Can you work these out from the model? Positions are in its coordinate system, mm. Face numbers are marked on the shaded views. A direction names the side the tool comes from. Give positions to 0.01 mm unless a question says otherwise; leave off trailing zeros. Order: outer loops, then holes, each group sorted by start corner. A loop starts at its lowest first (then second) coordinate and runs counter-clockwise, first axis right, second up. Notation, with made-up numbers: (-14.75, 4.25) - (18.25, 4.25) arc R21 ccw to (18.25, 32.25) - close; hole circle Ø2 at (77, 52.5). An arc over 180 degrees is marked (long way). Answer as a JSON object with one key per item and string values.
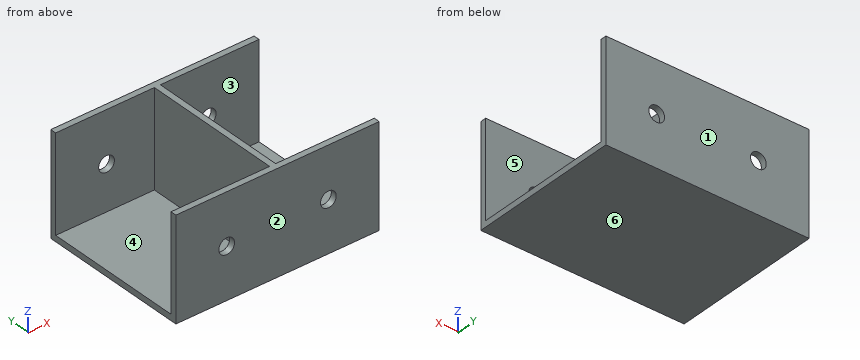
```python
from build123d import *

# Parameters (mm, degrees)
SKETCH1_W           = 101.6
SKETCH1_H           = 76.2
BOSS_EXTRUDE1_DEPTH = 50.8
SKETCH3_W           = 49.3
SKETCH3_H           = 70.2
CUT_EXTRUDE1_DEPTH  = 47.8
SKETCH4_R           = 3.937
CUT_EXTRUDE3_DEPTH  = 50.8


with BuildPart() as part:
    # Sketch1 → Boss-Extrude1 (new body)
    with BuildSketch(Plane.XY):
        Rectangle(SKETCH1_W, SKETCH1_H)
    extrude(amount=BOSS_EXTRUDE1_DEPTH)

    # Sketch3 → Cut-Extrude1 (cut)
    with BuildSketch(Plane.XY.offset(50.8)):
        with Locations((-26.15, 0)):
            Rectangle(SKETCH3_W, SKETCH3_H)
        with Locations((26.15, 0)):
            Rectangle(SKETCH3_W, SKETCH3_H)
    extrude(amount=-CUT_EXTRUDE1_DEPTH, mode=Mode.SUBTRACT)

    # Sketch4 → Cut-Extrude3 (cut, symmetric)
    with BuildSketch(Plane(origin=(0, 0, 0), x_dir=(1, 0, 0), z_dir=(0, 1, 0))):
        with Locations(Location((25.4, -25.4, 0), (0, 0, 270))):
            Circle(SKETCH4_R)
        with Locations(Location((-25.4, -25.4, 0), (0, 0, 270))):
            Circle(SKETCH4_R)
    extrude(amount=CUT_EXTRUDE3_DEPTH, both=True, mode=Mode.SUBTRACT)


solid = part.part
```
Q1. Which directions (+Z, -Z, +X, -X, +Y, -Y) give clear straight access to the entire face, cutting with the end or side of a thin tool? Please do the marked faces 4, 5 and 6.
Recorded:
{"face 4": "+Z, -X", "face 5": "+Z, +X", "face 6": "-Z, +X, -X, +Y, -Y"}
Q2. I'm going to push flat-ended pins straight in: pin 1 Ø10 at (x, y) = (-19.5, -2.5) entering from +Z; pin 2 Ø5 at (x, y) = (15, 4) entering from -Z; pin 3 Ø10 at (y, z) = (24, 13.5) entering from +X; pin 4 Ø14.5 at (y, z) = (0, 30.5) entering from -X. Where does each tip first touch, or does it pass through?
Recorded:
{"pin 1": "stops at z = 3", "pin 2": "stops at z = 0", "pin 3": "stops at x = 1.5", "pin 4": "stops at x = -1.5"}
Q3. If we section it at D-D, the plane x = 38: Please give me the cut outline in (y, z), then the cut area to 3 significant figures.
Recorded:
{"outline": "(-38.1, 0) - (38.1, 0) - (38.1, 50.8) - (35.1, 50.8) - (35.1, 3) - (-35.1, 3) - (-35.1, 50.8) - (-38.1, 50.8) - close", "area": "515 mm^2"}
Q4. I need wall thicknesses on L1, parallel to X at y = -37, z = 25; L2, parallel to Z at x = 25, y = -36; L3, parallel to Y at x = -19.5, z = 30. Which ranges of each line are inside material? Lowest first, please.
Recorded:
{"L1": "x = -50.8 to -29.32, -21.48 to 21.48, 29.32 to 50.8", "L2": "z = 0 to 21.48, 29.32 to 50.8", "L3": "y = -38.1 to -35.1, 35.1 to 38.1"}
Q5. If we section it at A-A, the plane z = 25.4: Please give me the cut outline in (x, y), then the cut area to 3 significant figures.
Recorded:
{"outline": "(-50.8, -38.1) - (-29.34, -38.1) - (-29.34, -35.1) - (-50.8, -35.1) - close; (-50.8, 35.1) - (-29.34, 35.1) - (-29.34, 38.1) - (-50.8, 38.1) - close; (-21.46, -38.1) - (21.46, -38.1) - (21.46, -35.1) - (1.5, -35.1) - (1.5, 35.1) - (21.46, 35.1) - (21.46, 38.1) - (-21.46, 38.1) - (-21.46, 35.1) - (-1.5, 35.1) - (-1.5, -35.1) - (-21.46, -35.1) - close; (29.34, -38.1) - (50.8, -38.1) - (50.8, -35.1) - (29.34, -35.1) - close; (29.34, 35.1) - (50.8, 35.1) - (50.8, 38.1) - (29.34, 38.1) - close", "area": "726 mm^2"}
Q6. If we section it at B-B, the plane x = 25.4: Please give me the cut outline in (y, z), then the cut area to 3 significant figures.
Recorded:
{"outline": "(-38.1, 0) - (38.1, 0) - (38.1, 21.46) - (35.1, 21.46) - (35.1, 3) - (-35.1, 3) - (-35.1, 21.46) - (-38.1, 21.46) - close; (-38.1, 29.34) - (-35.1, 29.34) - (-35.1, 50.8) - (-38.1, 50.8) - close; (35.1, 29.34) - (38.1, 29.34) - (38.1, 50.8) - (35.1, 50.8) - close", "area": "468 mm^2"}
Q7. If we section it at C-C, the plane y = 20.5: Please give me the cut outline in (x, z).
Recorded:
{"outline": "(-50.8, 0) - (50.8, 0) - (50.8, 3) - (1.5, 3) - (1.5, 50.8) - (-1.5, 50.8) - (-1.5, 3) - (-50.8, 3) - close"}
Q8. We'd pull the mould along Y, two halves only. Please class the marked faces 1, 2 and 3: released by +Y, released by -Y, zero draft, split by the parting line, or undercut.
Recorded:
{"face 1": "released by +Y", "face 2": "released by -Y", "face 3": "undercut"}
